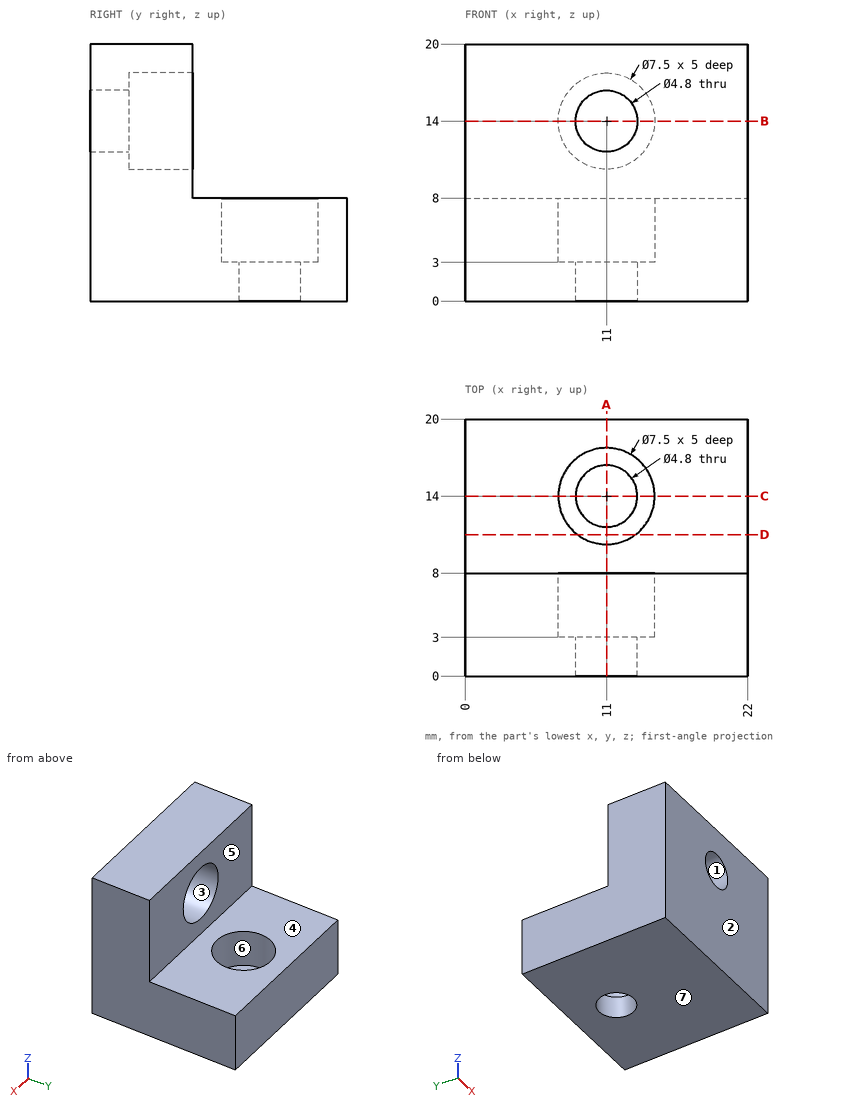
Geometry: see drawing. Coordinates: mm, zero at the bounding-box minimum. A direction names the side the tool comes from. Round coordinates to 2 decimals unless told otherwise and drop trailing zeros. Loops run counter-clockwise (first coordinate to the right, second up) from the corner with the lowest first, then second, coordinate; pieces in that order, holes last. Notation, with made-up numbers: M 50,-31 L 64,-31 A25 cw 64,3 Z; hole C -10,-2 d3. An arc over 180 degrees is marked long. Use a Markdown table: item, result. Add a question column.
1. Reachability of the marked faces 5, 6 and 7 from +Z, -Z, +X, -X, +Y, -Y: full face, straight path, thin tool, end or side. Return the list, or none.
2. Line query: line 1 (X direction, y = 6.15, z = 14); line 2 (Y direction, x = 11, z = 2.1); line 3 (Y direction, x = 2.5, z = 16.5). Output: solid intervals per line, ascending.
3. Section query A-A on x = 11. Return the cut outline in (y, z), then the cut area to 3 significant figures.
4. Section query B-B on z = 14. Return the cut outline in (x, y).
5. Section query D-D on y = 11. Return the cut outline in (x, z).
6. Mould query, pull axis Z, two halves, no side actions, for the marked faces 1, 2, 3 and 4. Classes: pulls with the +Z half, pulls with the -Z half, needs draft (parallel to the pull), parting line crosses it, or undercut.
7. Contact query for flat-ended pins moving along their axis: P1, Ø3, axis at x = 8, z = 18, coming from the +Y side; P2, Ø6, axis at x = 11, z = 14, coming from the +Y side; P3, Ø6, axis at x = 9.5, y = 12.5, coming from the +Z side. Output: stop coordinate, or through.
Reported:
| question | item | result |
|---|---|---|
| 1 | face 5 | +Z, +X, -X, +Y |
| 1 | face 6 | +Z |
| 1 | face 7 | -Z, +X, -X, +Y, -Y |
| 2 | line 1 | x = 0 to 7.25, 14.75 to 22 |
| 2 | line 2 | y = 0 to 11.6, 16.4 to 20 |
| 2 | line 3 | y = 0 to 8 |
| 3 | outline | M 0,0 L 11.6,0 L 11.6,3 L 10.25,3 L 10.25,8 L 8,8 L 8,10.25 L 3,10.25 L 3,11.6 L 0,11.6 Z; M 0,16.4 L 3,16.4 L 3,17.75 L 8,17.75 L 8,20 L 0,20 Z; M 16.4,0 L 20,0 L 20,8 L 17.75,8 L 17.75,3 L 16.4,3 Z |
| 3 | area | 152 mm² |
| 4 | outline | M 0,0 L 8.6,0 L 8.6,3 L 7.25,3 L 7.25,8 L 0,8 Z; M 13.4,0 L 22,0 L 22,8 L 14.75,8 L 14.75,3 L 13.4,3 Z |
| 5 | outline | M 0,0 L 22,0 L 22,8 L 13.25,8 L 13.25,3 L 8.75,3 L 8.75,8 L 0,8 Z |
| 6 | face 1 | undercut |
| 6 | face 2 | needs draft |
| 6 | face 3 | undercut |
| 6 | face 4 | pulls with the +Z half |
| 7 | P1 | stops at y = 8 |
| 7 | P2 | stops at y = 3 |
| 7 | P3 | stops at z = 8 |
